from build123d import *

# Parameters (mm, degrees)
SALIENTE_EXTRUIR2_DEPTH = 100
CORTAR_EXTRUIR1_DEPTH   = 100
REDONDEO1_R             = 12
REDONDEO2_R             = 12


with BuildPart() as part:
    # Croquis1 → Saliente-Extruir2 (new body)
    with BuildSketch(Plane(origin=(0, 0, 0), x_dir=(1, 0, 0), z_dir=(0, 1, 0))):
        Polygon((-50, -86.602540378), (50, -86.602540378), (100, 0), (50, 86.602540378), (-50, 86.602540378), (-100, 0), align=None)
    extrude(amount=SALIENTE_EXTRUIR2_DEPTH)

    # Croquis3 → Cortar-Extruir1 (cut)
    with BuildSketch(Plane(origin=(0, 100, 0), x_dir=(1, 0, 0), z_dir=(0, 1, 0))):
        Polygon((39.613585437, -69.686093894), (80.156720321, -0.536675623), (40.543134884, 69.14941827), (-39.613585437, 69.686093894), (-80.156720321, 0.536675623), (-40.543134884, -69.14941827), align=None)
    extrude(amount=-CORTAR_EXTRUIR1_DEPTH, mode=Mode.SUBTRACT)

    # Redondeo1
    redondeo1_edges = [part.edges().sort_by_distance(p)[0] for p in [
        (-100, 50, 0),
        (-50, 50, -86.602540378),
        (50, 50, -86.602540378),
        (100, 50, 0),
        (50, 50, 86.602540378),
        (-50, 50, 86.602540378),
    ]]
    fillet(redondeo1_edges, radius=REDONDEO1_R)

    # Redondeo2
    redondeo2_edges = [part.edges().sort_by_distance(p)[0] for p in [
        (39.613585437, 50, 69.686093894),
        (-40.543134884, 50, 69.14941827),
        (-80.156720321, 50, -0.536675623),
        (-39.613585437, 50, -69.686093894),
        (40.543134884, 50, -69.14941827),
        (80.156720321, 50, 0.536675623),
    ]]
    fillet(redondeo2_edges, radius=REDONDEO2_R)


solid = part.part
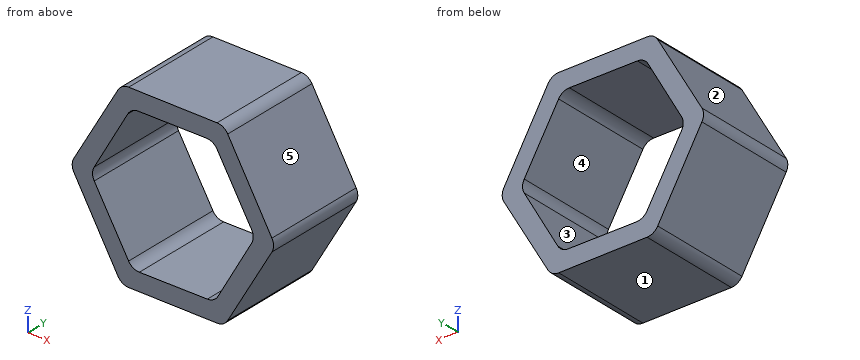
Geometry: final body of the model. Coordinates: model frame, mm. Face numbers are marked on the shaded views. A direction names the side the tool comes from. Round coordinates to 2 decimals unless told otherwise and drop trailing zeros. Order: outer loops, then holes, each group sorted by start corner. A loop starts at its lowest first (then second) coordinate and runs counter-clockwise, first axis right, second up.
Q1. Section A-A, the plane x = 40.5. Output: boundary loops of the cut face in (y, z).
Result sheet:
outline: (0, -86.6) - (100, -86.6) - (100, -66.97) - (0, -66.97) - close; (0, 66.82) - (100, 66.82) - (100, 86.6) - (0, 86.6) - close
Q2. Access query for the marked faces 4 and 5. Directions: +Z, -Z, +X, -X, +Y, -Y. A direction counts if a zero-diameter tool reaches every point of the face in a straight line with its end or side. Return the directions, or none.
Result sheet:
face 4: +Y, -Y
face 5: +Z, +X, +Y, -Y
Q3. Section D-D, the plane z = 76. Output: boundary loops of the cut face in (x, y).
Result sheet:
outline: (-56.12, 0) - (56.12, 0) - (56.12, 100) - (-56.12, 100) - close
Q4. Material intervals for probe 1 along Z at (x, y) = (-30, 84); probe 2 along Z at (x, y) = (12.5, 72.5); probe 3 along X at (y, z) = (37, 52.5), sorted ascending.
Result sheet:
probe 1: z = -86.6 to -69.62, 69.22 to 86.6
probe 2: z = -86.6 to -69.34, 69.5 to 86.6
probe 3: x = -69.69 to -50.01, 49.69 to 69.69
Q5. Section C-C, the plane z = -23. Output: boundary loops of the cut face in (x, y).
Result sheet:
outline: (-86.72, 0) - (-66.99, 0) - (-66.99, 100) - (-86.72, 100) - close; (66.78, 0) - (86.72, 0) - (86.72, 100) - (66.78, 100) - close
Q6. Mould query, pull axis X, two halves, no side actions, for the marked faces 1, 2 and 3. Classes: released by +X, released by -X, zero draft, split by the parting line, or undercut.
Result sheet:
face 1: zero draft
face 2: released by -X
face 3: undercut
Q7. Section B-B, the plane y = 25. Output: boundary loops of the cut face in (x, z).
Result sheet:
outline: (-96.54, -6) - (-53.46, -80.6) arc R12 ccw to (-43.07, -86.6) - (43.07, -86.6) arc R12 ccw to (53.46, -80.6) - (96.54, -6) arc R12 ccw to (96.54, 6) - (53.46, 80.6) arc R12 ccw to (43.07, 86.6) - (-43.07, 86.6) arc R12 ccw to (-53.46, 80.6) - (-96.54, 6) arc R12 ccw to start; hole (-76.73, 5.49) arc R12 ccw to (-76.65, -6.51) - (-43.12, -63.71) arc R12 ccw to (-32.69, -69.64) - (33.62, -69.2) arc R12 ccw to (43.97, -63.13) - (76.73, -5.49) arc R12 ccw to (76.65, 6.51) - (43.12, 63.71) arc R12 ccw to (32.69, 69.64) - (-33.62, 69.2) arc R12 ccw to (-43.97, 63.13) - close
Q8. Pin query (flat end, axial travel): pin 1 (3 mm diameter, centred on x = -69, z = 35, fed in from -Y); pin 2 (10 mm diameter, centred on y = 75, z = -27, fed in from +X); pin 3 (2 mm diameter, centred on x = 72.5, y = 61.5, fed in from +Z); pin 4 (10 mm diameter, centred on x = 74.5, y = 19, fed in from +Z). Return the tip coordinate at first contact, or that it passes through.
Result sheet:
pin 1: stops at y = 0
pin 2: stops at x = 87.3
pin 3: stops at z = 49.36
pin 4: stops at z = 52.83
